Geometry check sheet. Reference: the model listing, model coordinates, mm. Face numbers are marked on the shaded views. A direction names the side the tool comes from. Coordinates: 2 decimals unless noted, no trailing zeros. Order: outer loops, then holes, each group sorted by start corner. A loop starts at its lowest first (then second) coordinate and runs counter-clockwise, first axis right, second up. Notation, with made-up numbers: (-10, 7) - (37, 7) arc R5 cw to (37, 15) - close; hole circle Ø5 at (74.5, 11). An arc over 180 degrees is marked (long way). Use CSV: the item, a comma, the result in double quotes. Start each with the question number.
1) Tool access check on the marked faces 1 and 2. Record the directions out of +Z, -Z, +X, -X, +Y, -Y that give a thin tool (end or side, any length) a straight path to the whole face; none if there is none.
2) Thickness scan on probe 1 along Y at (x, z) = (0, 39); probe 2 along X at (y, z) = (-0.25, 30.5); probe 3 along Z at (x, y) = (-2.5, 0.25). Record the ranges inside material, lowest first. Write a range as [from, to].
3) Depth check by flat-ended pin: P1, Ø1, axis at y = -0.5, z = 32.5, coming from the -X side; P2, Ø8, axis at x = 4, z = 70.5, coming from the -Y side; P3, Ø1, axis at y = 1.5, z = 36.5, coming from the -X side. Enter the tip coordinate at first touch or a pass-through.
4) Sectioned sample at A-A, the plane x = 0. Record the cut outline in (y, z), and give its area (3 significant figures).
Autodesk Inventor part; units mm, degrees
ref_plane "YZ Plane" through (0, 0, 0) normal (1, 0, 0) x (0, 1, 0)
ref_plane "XZ Plane" through (0, 0, 0) normal (0, 1, 0) x (-1, 0, 0)
ref_plane "XY Plane" through (0, 0, 0) normal (0, 0, 1) x (1, 0, 0)
sketch "Sketch1" plane through (0, 0, 0) normal (0, 0, 1) x (1, 0, 0)
  circle A0 centre (0, 0) radius 4
  dimension "Diameter" = 8
extrude "Extrusion1" add sketch "Sketch1" along normal blind 75.04
sketch "Sketch2" plane through (0, 0, 75.04) normal (0, 0, 1) x (1, 0, 0)
  circle A0 centre (0, 0) radius 4
extrude "Extrusion2" add sketch "Sketch2" along normal blind 4.96 draft 45
sketch "Sketch3" plane through (0, 0, 80) normal (0, 0, 1) x (1, 0, 0)
  circle A0 centre (0, 0) radius 8.96
  circle A1 centre (0, 0) radius 2.8868 construction
  line L0 (1.2084, 2.6217) -> (2.8746, 0.2644)
  line L1 (2.8746, 0.2644) -> (1.6662, -2.3573)
  line L2 (1.6662, -2.3573) -> (-1.2084, -2.6217)
  line L3 (-1.2084, -2.6217) -> (-2.8746, -0.2644)
  line L4 (-2.8746, -0.2644) -> (-1.6662, 2.3573)
  line L5 (-1.6662, 2.3573) -> (1.2084, 2.6217)
  dimension "Hex_Width" = 5
extrude "Extrusion3" cut sketch "Sketch3" against normal blind 3 contours L0 L1 L2 L3 L4 L5
thread "Thread1"
chamfer "Chamfer2" distance 0.8 angle 45 1 edges at (-4, 0, 0)
fillet "Fillet1" radius 0.1 1 edges at (-8.96, 0, 80)
equation "\"d10\" = Thread_Length"
equation "\"d13\" = Chamfer"
equation "\"Thread_Length\" = 45"
properties part number "SCREW,FLAT HD,P, 5,M8X1.25X80MM"
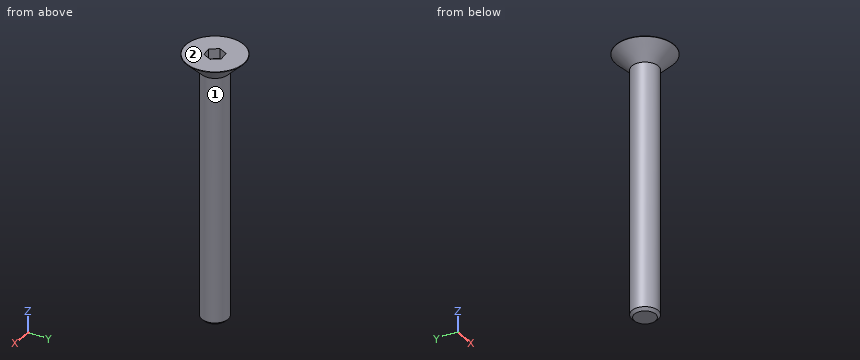
Evaluation:
1,face 1,"-Z"
1,face 2,"+Z, +X, -X, +Y, -Y"
2,probe 1,"[-4, 4]"
2,probe 2,"[-3.99, 3.99]"
2,probe 3,"[0, 77]"
3,P1,"x = -4"
3,P2,"y = -4"
3,P3,"x = -3.87"
4,outline,"(-8.79, 79.83) - (-4, 75.04) - (-4, 0.8) - (-3.2, 0) - (3.2, 0) - (4, 0.8) - (4, 75.04) - (8.79, 79.83) arc R0.1 ccw to (8.72, 80) - (2.51, 80) - (2.51, 77) - (-2.51, 77) - (-2.51, 80) - (-8.72, 80) arc R0.1 ccw to start"
4,area,"649 mm²"
